Autodesk Inventor part; units mm, degrees
ref_plane "YZ Plane" through (0, 0, 0) normal (1, 0, 0) x (0, 1, 0)
ref_plane "XZ Plane" through (0, 0, 0) normal (0, 1, 0) x (-1, 0, 0)
ref_plane "XY Plane" through (0, 0, 0) normal (0, 0, 1) x (1, 0, 0)
sketch "Sketch1" plane through (0, 0, 0) normal (0, 0, 1) x (1, 0, 0)
  line L0 (-12.1708, 16.0073) -> (13.2292, 16.0073)
  line L1 (13.2292, 16.0073) -> (13.2292, -34.7927)
  line L2 (13.2292, -34.7927) -> (-12.1708, -34.7927)
  line L3 (-12.1708, -34.7927) -> (-12.1708, 16.0073)
  line L4 (11.9592, 14.7373) -> (-10.9008, 14.7373)
  line L5 (-10.9008, 14.7373) -> (-10.9008, -33.5227)
  line L6 (-10.9008, -33.5227) -> (11.9592, -33.5227)
  line L7 (11.9592, -33.5227) -> (11.9592, 14.7373)
  point P0 (0, 0)
  dimension "d0" = 25.4
  dimension "d1" = 50.8
  dimension "d2" = 1.27
extrude "Extrusion1" add sketch "Sketch1" along normal blind 152.4
sketch "Sketch2" plane through (-12.1708, 16.0073, 0) normal (0, 1, 0) x (1, 0, 0)
  circle A0 centre (12.7, -12.7) radius 1.7272
  line L0 (25.4, 0) -> (0, 0)
  line L1 (0, 0) -> (0, -152.4)
  point P0 (12.1708, 0)
  dimension "d5" = 3.4544
  dimension "d6" = 12.7
  dimension "d7" = 12.7
extrude "Extrusion2" cut sketch "Sketch2" against normal through all
pattern_linear "Rectangular Pattern1" count 6 spacing 25.4 along (0, 0, 1) of "Extrusion2"
equation "\"d3\" = d13"
equation "\"d13\" = 152.4"
properties part number "VerseFrame 6in"
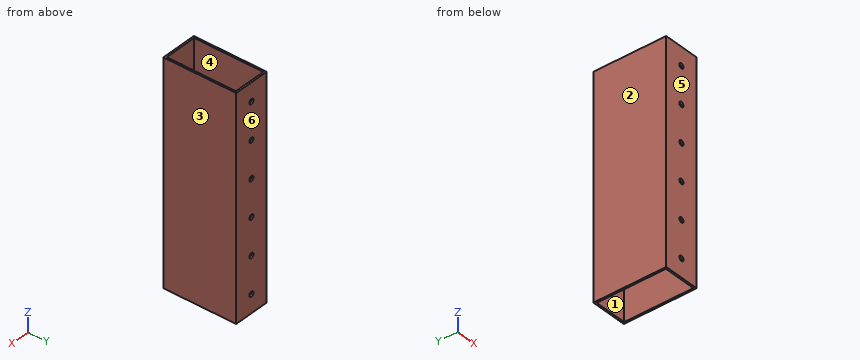
For this review, take the finished solid that the model builds, in its own axes (mm). Face numbers are marked on the shaded views. A direction names the side the tool comes from. Round coordinates to 2 decimals unless told otherwise and drop trailing zeros. Loops run counter-clockwise (first coordinate to the right, second up) from the corner with the lowest first, then second, coordinate; pieces in that order, holes last. Notation, with made-up numbers: (38.5, 67) - (43.5, 67) arc R24 cw to (43.5, 91) - close; hole circle Ø11 at (3, 78). An arc over 180 degrees is marked (long way). One line per item, written item: value. Start each with the question number.
Item 1: Take a section at D-D (z = 63.5). Give the boundary of the cut face in (x, y).
Item 2: Take a section at A-A (y = -13). Give the boundary of the cut face in (x, z), plus the area to 3 significant figures.
Item 3: Take a section at C-C (z = 134). Give the boundary of the cut face in (x, y), plus the area to 3 significant figures.
Item 4: Take a section at B-B (x = -6.25). Give the boundary of the cut face in (y, z), plus the area to 3 significant figures.
Item 5: The part is to be moulded in two halves that separate along Y. For the marked faces 3, 4, 5 and 6, say which applies: +Y half, -Y half, draft (parallel to the pull), parting line (faces both ways), or undercut.
Item 6: For L1, parallel to X at y = 15.15, z = 139.7; L2, parallel to X at y = 1, z = 101; L3, parallel to Y at x = -4.25, z = 31, list the stretches that pass through material, from the lowest coordinate up.
Item 7: Clearance check with a flat-ended pin moving along its axis: pin 1 Ø2 at (x, z) = (0.53, 12.7) entering from +Y. State where the tip first meets the part, or that it passes through.
Item 8: For the marked faces 1 and 2, list the 3-axis set-ups (+Z, -Z, +X, -X, +Y, -Y) from which the entire face can be reached by the end or side of a thin tool; tool diameter is ignored.
Answer below:
1. outline: (-12.17, -34.79) - (-1.2, -34.79) - (-1.2, -33.52) - (-10.9, -33.52) - (-10.9, 14.74) - (-1.2, 14.74) - (-1.2, 16.01) - (-12.17, 16.01) - close; (2.26, -34.79) - (13.23, -34.79) - (13.23, 16.01) - (2.26, 16.01) - (2.26, 14.74) - (11.96, 14.74) - (11.96, -33.52) - (2.26, -33.52) - close
2. outline: (-12.17, 0) - (-10.9, 0) - (-10.9, 152.4) - (-12.17, 152.4) - close; (11.96, 0) - (13.23, 0) - (13.23, 152.4) - (11.96, 152.4) - close
2. area: 387 mm2
3. outline: (-12.17, -34.79) - (13.23, -34.79) - (13.23, 16.01) - (-12.17, 16.01) - close; hole (-10.9, -33.52) - (11.96, -33.52) - (11.96, 14.74) - (-10.9, 14.74) - close
3. area: 187 mm2
4. outline: (-34.79, 0) - (-33.52, 0) - (-33.52, 152.4) - (-34.79, 152.4) - close; (14.74, 0) - (16.01, 0) - (16.01, 152.4) - (14.74, 152.4) - close
4. area: 387 mm2
5. face 3: draft
5. face 4: undercut
5. face 5: -Y half
5. face 6: +Y half
6. L1: x = -12.17 to -1.2, 2.26 to 13.23
6. L2: x = -12.17 to -10.9, 11.96 to 13.23
6. L3: y = -34.79 to -33.52, 14.74 to 16.01
7. pin 1: passes through
8. face 1: +Z, -Z
8. face 2: +Z, -Z, -X, +Y, -Y
